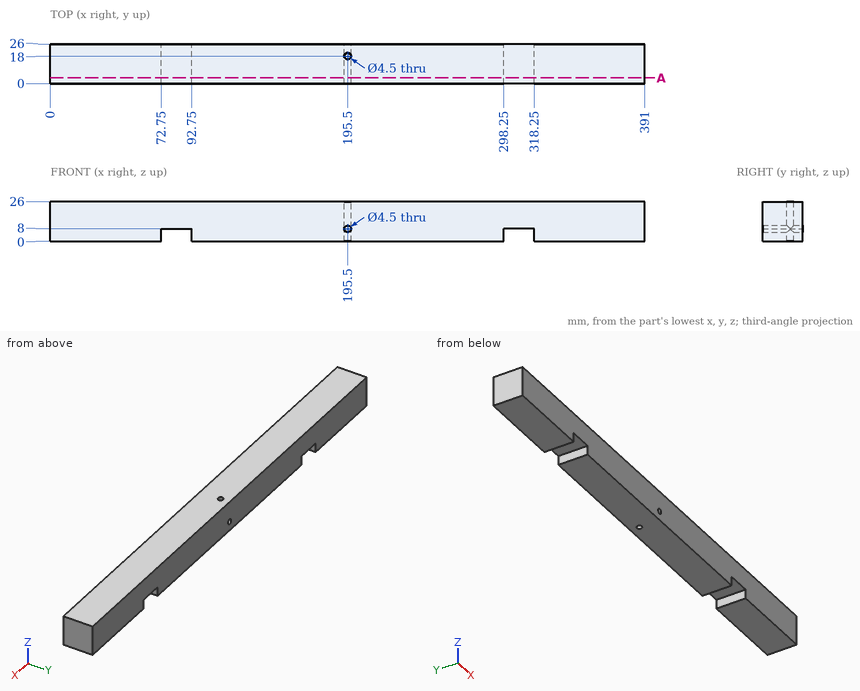
The figure shows three views and two pictorial views of one solid part (mm, origin at its lowest corner). Answer the questions. Round coordinates to 2 decimals unless told otherwise and drop trailing zeros. Loops run counter-clockwise (first coordinate to the right, second up) from the corner with the lowest first, then second, coordinate; pieces in that order, holes last. Notation, with made-up numbers: M -12,52.25 L 38,52.25 A17 ccw 38,80.25 Z; hole C -33.75,84 d4. An arc over 180 degrees is marked long. Use CSV: the item, a comma, the result in double quotes.
Q1. Each of these flat-tipped pins is pushed along its axis until it touches: pin 1 (10 mm diameter, centred on x = 86, y = 13, fed in from -Z); pin 2 (2.5 mm diameter, centred on x = 195.5, y = 18, fed in from -Z). Where does it stop, or does it pass through?
Determined:
pin 1,"z = 8"
pin 2,"through"
Q2. Consider L1, parallel to X at y = 15.5, z = 4.25; L2, parallel to X at y = 18, z = 3.5; L3, parallel to Y at x = 195.5, z = 21.5. Determine where each line is inside the solid, lowest interval first.
Determined:
L1,"0 to 72.75, 92.75 to 298.25, 318.25 to 391"
L2,"0 to 72.75, 92.75 to 193.25, 197.75 to 298.25, 318.25 to 391"
L3,"0 to 15.75, 20.25 to 26"
Q3. Section A-A, the plane y = 3.75 is taken. Determine the outline of the cut face in (x, z), then the cut area to 3 significant figures.
Determined:
outline,"M 0,0 L 72.75,0 L 72.75,8 L 92.75,8 L 92.75,0 L 298.25,0 L 298.25,8 L 318.25,8 L 318.25,0 L 391,0 L 391,26 L 0,26 Z; hole C 195.5,8 d4.5"
area,"9,830 mm2"
